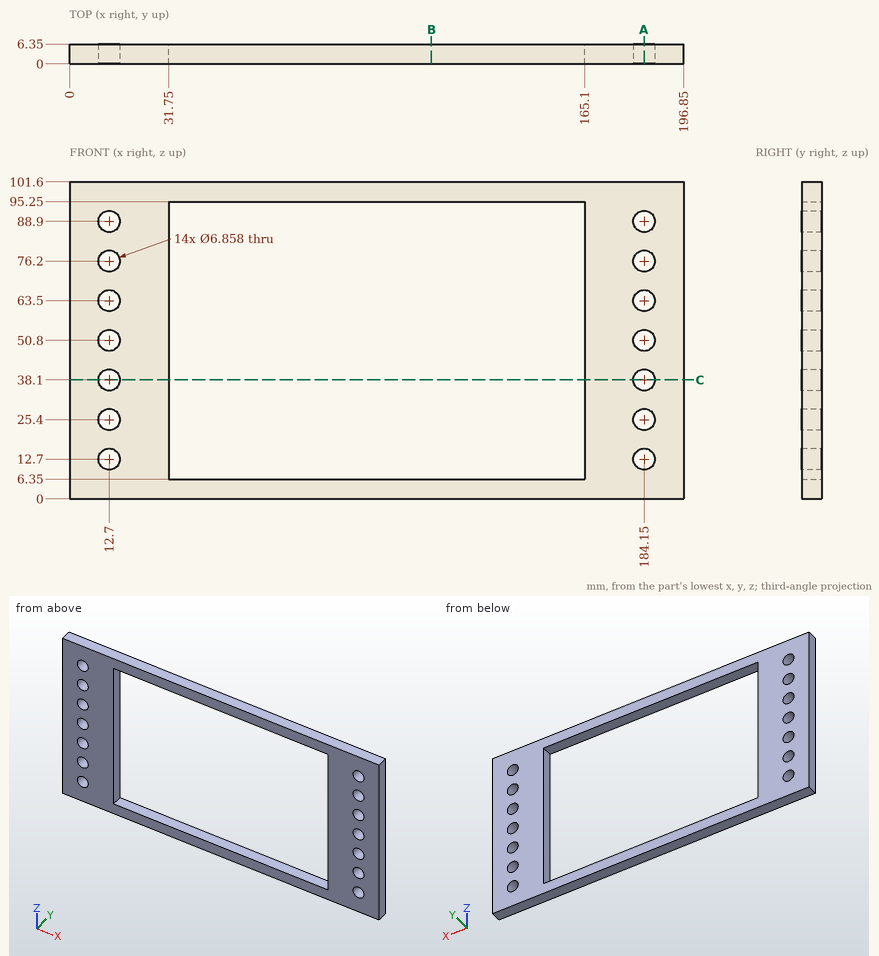
Can you work these out from the drawing? Everything is in mm from the part's minimum corner. Give positions to 0.01 mm unless a question says otherwise; leave off trailing zeros. Order: outer loops, then holes, each group sorted by start corner. A loop starts at its lowest first (then second) coordinate and runs counter-clockwise, first axis right, second up.
1. I need wall thicknesses on L1, parallel to X at y = 3.5, z = 50.8; L2, parallel to Z at x = 44, y = 0.5; L3, parallel to X at y = 1.5, z = 14.5. Which ranges of each line are inside material? Lowest first, please.
2. Suppose I cut it at A-A (x = 184.15). Give the number of separate pieces and of enclosed holes in the cut face, plus the area to 3 significant figures.
3. Suppose I cut it at C-C (z = 38.1). List the corners of the cut face in (x, y) for me, plus the area to 3 significant figures.
4. Suppose I cut it at B-B (x = 116). List the corners of the cut face in (y, z) for me.
Solved:
1. L1: x = 0 to 9.27, 16.13 to 31.75, 165.1 to 180.72, 187.58 to 196.85
1. L2: z = 0 to 6.35, 95.25 to 101.6
1. L3: x = 0 to 9.78, 15.62 to 31.75, 165.1 to 181.23, 187.07 to 196.85
2. separate pieces: 8
2. enclosed holes: 0
2. area: 340 mm2
3. outline: (0, 0) - (9.27, 0) - (9.27, 6.35) - (0, 6.35) - close; (16.13, 0) - (31.75, 0) - (31.75, 6.35) - (16.13, 6.35) - close; (165.1, 0) - (180.72, 0) - (180.72, 6.35) - (165.1, 6.35) - close; (187.58, 0) - (196.85, 0) - (196.85, 6.35) - (187.58, 6.35) - close
3. area: 316 mm2
4. outline: (0, 0) - (6.35, 0) - (6.35, 6.35) - (0, 6.35) - close; (0, 95.25) - (6.35, 95.25) - (6.35, 101.6) - (0, 101.6) - close
